Verification items for the finished model (mm, model axes). Round coordinates to 2 decimals unless told otherwise and drop trailing zeros. Write each loop counter-clockwise with the first axis right and the second up, starting at its lowest first coordinate (ties: lowest second). Pieces come first, ordered by that corner, then holes. Notation, with made-up numbers: (64.25, 37.5) -> (87.25, 37.5) arc R27 cw to (87.25, 54.5) -> close; hole circle Ø9 at (12.25, -25). An arc over 180 degrees is marked (long way). Use CSV: the item, a comma, the result in double quotes.
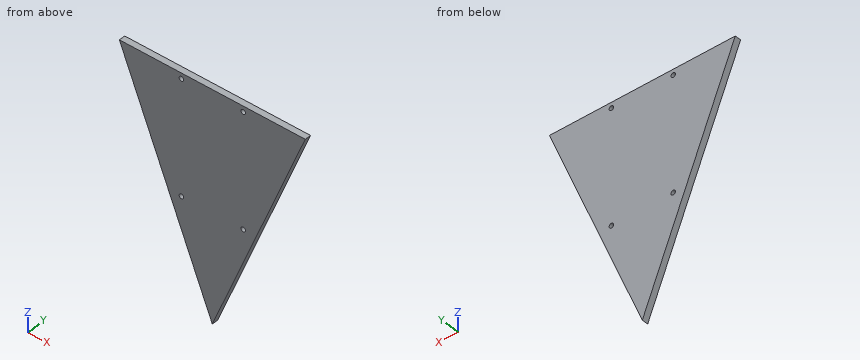
```python
from build123d import *

# Parameters (mm, degrees)
SKETCH1_R           = 2
BOSS_EXTRUDE1_DEPTH = 5
SKETCH3_W           = 64.166552172
SKETCH3_H           = 97.438097742
BOSS_EXTRUDE2_DEPTH = 5
SKETCH4_R           = 1.825
CUT_EXTRUDE1_DEPTH  = 10


with BuildPart() as part:
    # Sketch1 → Boss-Extrude1 (new body)
    with BuildSketch(Plane(origin=(0, 0, 0), x_dir=(1, 0, 0), z_dir=(0, 1, 0))):
        Polygon((75.179761571, 0), (0, 181.5), (-75.179761571, 0), align=None)
        with Locations((27.701843901, 4.378893659)):
            Circle(SKETCH1_R, mode=Mode.SUBTRACT)
        with Locations((-27.701843901, 4.378893659)):
            Circle(SKETCH1_R, mode=Mode.SUBTRACT)
        with Locations((-27.701843901, 95.621106341)):
            Circle(SKETCH1_R, mode=Mode.SUBTRACT)
        with Locations((27.701843901, 95.621106341)):
            Circle(SKETCH1_R, mode=Mode.SUBTRACT)
    extrude(amount=BOSS_EXTRUDE1_DEPTH)

    # Sketch3 → Boss-Extrude2 (add)
    with BuildSketch(Plane(origin=(0, 5, 0), x_dir=(1, 0, 0), z_dir=(0, 1, 0))):
        with Locations((-0.392642939, 50.723354507)):
            Rectangle(SKETCH3_W, SKETCH3_H)
    extrude(amount=-BOSS_EXTRUDE2_DEPTH)

    # Sketch4 → Cut-Extrude1 (cut)
    with BuildSketch(Plane(origin=(0, 5, 0), x_dir=(1, 0, 0), z_dir=(0, 1, 0))):
        with Locations((-25, 4.5)):
            Circle(SKETCH4_R)
        with Locations((25, 4.5)):
            Circle(SKETCH4_R)
        with Locations((25, 95.5)):
            Circle(SKETCH4_R)
        with Locations((-25, 95.5)):
            Circle(SKETCH4_R)
    extrude(amount=-CUT_EXTRUDE1_DEPTH, mode=Mode.SUBTRACT)


solid = part.part
```
Q1. Section check A-A (y = 2.95). Record the cut outline in (x, z) (3 decimals), plus the area to 3 significant figures.
Filled in:
outline,"(-75.18, 0) -> (0, -181.5) -> (75.18, 0) -> close; hole circle Ø3.65 at (-25, -95.5); hole circle Ø3.65 at (-25, -4.5); hole circle Ø3.65 at (25, -95.5); hole circle Ø3.65 at (25, -4.5)"
area,"13,600 mm²"
Q2. Material ranges on L1, parallel to Z at x = -25, y = 2.55 (3 decimals); L2, parallel to X at y = 1.1, z = -4.5 (3 decimals); L3, parallel to Z at x = -68, y = 4.25, recorded low to high.
Filled in:
L1,"-121.145 to -97.325, -93.675 to -6.325, -2.675 to 0"
L2,"-73.316 to -26.825, -23.175 to 23.175, 26.825 to 73.316"
L3,"-17.33 to 0"
Q3. Section check B-B (z = -59). Record the cut outline in (x, y), plus the area to 3 significant figures.
Filled in:
outline,"(-50.74, 0) -> (50.74, 0) -> (50.74, 5) -> (-50.74, 5) -> close"
area,"507 mm²"
Q4. Section check C-C (x = 60). Record the cut outline in (y, z).
Filled in:
outline,"(0, -36.65) -> (5, -36.65) -> (5, 0) -> (0, 0) -> close"
Q5. Go/stop test with flat-tipped pins: P1, Ø1, axis at x = 6, y = 2, coming from the -Z side; P2, Ø3, axis at x = -43, y = 2, coming from the -Z side. Record where each tip stops, or that it passes through.
Filled in:
P1,"z = -168.22"
P2,"z = -81.31"
